from build123d import *

# Parameters (mm, degrees)
SKETCH1_W                                        = 203.2
SKETCH1_H                                        = 203.2
BOSS_EXTRUDE1_DEPTH                              = 25.4
CBORE_FOR_1_4_SOCKET_HEAD_CAP_SCREW1_D           = 6.7564
CBORE_FOR_1_4_SOCKET_HEAD_CAP_SCREW1_CBORE_D     = 11.1125
CBORE_FOR_1_4_SOCKET_HEAD_CAP_SCREW1_CBORE_DEPTH = 18.3500014
CBORE_FOR_3_8_SOCKET_HEAD_CAP_SCREW1_D           = 10.0838
CBORE_FOR_3_8_SOCKET_HEAD_CAP_SCREW1_CBORE_D     = 15.875
CBORE_FOR_3_8_SOCKET_HEAD_CAP_SCREW1_CBORE_DEPTH = 9.525


with BuildPart() as part:
    # Sketch1 → Boss-Extrude1 (new body)
    with BuildSketch(Plane(origin=(0, 0, 0), x_dir=(1, 0, 0), z_dir=(0, 1, 0))):
        with Locations((101.6, 101.6)):
            Rectangle(SKETCH1_W, SKETCH1_H)
    extrude(amount=BOSS_EXTRUDE1_DEPTH)

    # CBORE for 1/4 Socket Head Cap Screw1 (through all)
    with Locations(Plane(origin=(0, 0, 0), x_dir=(-1, 0, 0), z_dir=(0, -1, 0))):
        with Locations((-144.4625, 64.135), (-58.7375, 61.595), (-58.7375, 141.605), (-144.4625, 137.795)):
            CounterBoreHole(CBORE_FOR_1_4_SOCKET_HEAD_CAP_SCREW1_D / 2, CBORE_FOR_1_4_SOCKET_HEAD_CAP_SCREW1_CBORE_D / 2, CBORE_FOR_1_4_SOCKET_HEAD_CAP_SCREW1_CBORE_DEPTH)

    # CBORE for 3/8 Socket Head Cap Screw1 (through all)
    with Locations(Plane(origin=(0, 25.4, 0), x_dir=(1, 0, 0), z_dir=(0, 1, 0))):
        with Locations((29.718, 173.482), (29.718, 29.718), (173.482, 29.718), (173.482, 173.482)):
            CounterBoreHole(CBORE_FOR_3_8_SOCKET_HEAD_CAP_SCREW1_D / 2, CBORE_FOR_3_8_SOCKET_HEAD_CAP_SCREW1_CBORE_D / 2, CBORE_FOR_3_8_SOCKET_HEAD_CAP_SCREW1_CBORE_DEPTH)


solid = part.part
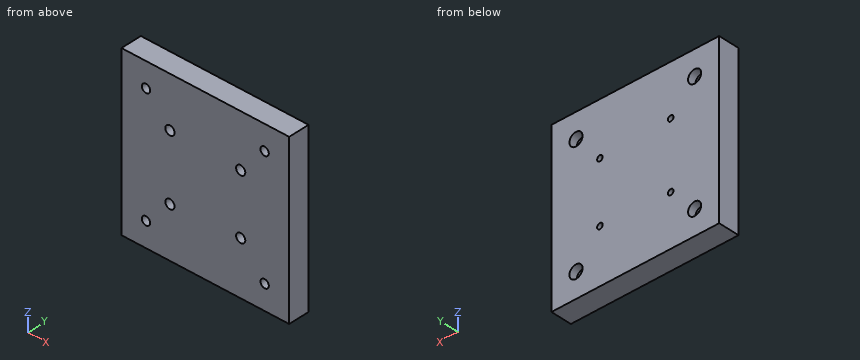
Source: CAD feature listing. Evaluate the final solid. Frame: model axes, mm. Give positions to 0.01 mm unless a question says otherwise; leave off trailing zeros. Write item = value, one per line. Start each with the question number.
Q1. Pin query (flat end, axial travel): pin 1 Ø8 at (x, z) = (33.5, -173.5) entering from +Y (3 decimals); pin 2 Ø3.5 at (x, z) = (146, -62) entering from -Y; pin 3 Ø6 at (x, z) = (29.718, -173.482) entering from -Y. Return the tip coordinate at first contact, or that it passes through.
Q2. Material intervals for probe 1 along X at (y, z) = (23.75, -26.5); probe 2 along X at (y, z) = (3.25, -176.5); probe 3 along Z at (x, y) = (31.5, 6.5), sorted ascending.
Q3. Cut plane A-A, the plane y = 4.75. Give the number of separate pieces and of enclosed holes in the cut face, then the cut area to 3 significant figures.
Computed values:
q1.pin_1 = 15.875
q1.pin_2 = 18.35
q1.pin_3 = through
q2.probe_1 = 0 to 22.46, 36.97 to 166.23, 180.74 to 203.2
q2.probe_2 = 0 to 25.68, 33.76 to 169.44, 177.52 to 203.2
q2.probe_3 = -203.2 to -178.2, -168.77 to -34.43, -25 to 0
q3.separate_pieces = 1
q3.enclosed_holes = 8
q3.area = 40,600 mm²
